Model file for the job. Use its own axes, mm. A direction names the side the tool comes from. Round coordinates to 2 decimals unless told otherwise and drop trailing zeros. Order: outer loops, then holes, each group sorted by start corner. A loop starts at its lowest first (then second) coordinate and runs counter-clockwise, first axis right, second up. Notation, with made-up numbers: M -16.75,-14 L 29.25,-14 A13 cw 29.25,-1 Z; hole C 2.25,-40 d2. An arc over 180 degrees is marked long. Return JSON: item names as keys, results as strings. Group by question number.
Item 1: Slice it at A-A on z = -24. Write the cut outline in (x, y).
Item 2: Pull direction Z, two halves, no side cores. Call faces 1 (the face through (13, 13.839, -13)), 2 (the face through (15.62, 21.51, -3.47)), 3 (the face through (-1.32, 25.33, -29.97)): pulls with the +Z half, pulls with the -Z half, needs draft (parallel to the pull), parting line crosses it, or undercut.
Item 3: Probe line 1 along Z through (x, y) = (0, 24.75); line 2 along X through (y, z) = (27.75, 7). List the from-to ranges inside material, lowest first.
Item 4: Which spindle directions (+Z, -Z, +X, -X, +Y, -Y) get a long thin tool onto all of the face, cutting with end or side? Do faces 4 (the face through (13, 25.839, -13)), 5 (the face through (-1.32, 13.33, -29.97)). Say none if no direction does.
Item 5: Slice it at B-B on y = 23. Write the cut outline in (x, z).
Item 6: Pin check, flat tips, straight feed: pin 1 Ø3 at (x, y) = (-20, 30.5) entering from -Z; pin 2 Ø12 at (y, z) = (12.5, -14) entering from -X; pin 3 Ø3 at (x, y) = (14, 24) entering from -Z. Stop position of each tip, or through.
from build123d import *

# Parameters (mm, degrees)
LPATTERN1_COUNT    = 7
LPATTERN1_PITCH    = 4
SKETCH3_R          = 19.047367533
CUT_EXTRUDE3_DEPTH = 4


with BuildPart() as part:
    # Sketch1 → Revolve1 (revolve)
    with BuildSketch(Plane(origin=(0, 0, 0), x_dir=(0, 0, -1), z_dir=(1, 0, 0))):
        Polygon((-18, 13.838658872), (-18, 9.838658872), (-30, 9.838658872), (-30, 8.838658872), (-16, 8.838658872), (-16, 13.838658872), align=None)
    revolve1 = revolve(axis=Axis((0, 28.058626224, 0), (0, -1, 0)))

    # LPattern1: Revolve1 ×7
    with Locations(*[(0, i * LPATTERN1_PITCH, 0) for i in range(1, LPATTERN1_COUNT)]):
        add(revolve1)

    # Sketch3 → Cut-Extrude3 (cut)
    with BuildSketch(Plane(origin=(0, 37.838658872, 0), x_dir=(1, 0, 0), z_dir=(0, 1, 0))):
        Circle(SKETCH3_R)
    extrude(amount=-CUT_EXTRUDE3_DEPTH, mode=Mode.SUBTRACT)


solid = part.part
Output values:
{
 "1": {"outline": "M -18,8.84 L 18,8.84 L 18,9.84 L -18,9.84 Z; M -18,12.84 L 18,12.84 L 18,13.84 L -18,13.84 Z; M -18,16.84 L 18,16.84 L 18,17.84 L -18,17.84 Z; M -18,20.84 L 18,20.84 L 18,21.84 L -18,21.84 Z; M -18,24.84 L 18,24.84 L 18,25.84 L -18,25.84 Z; M -18,28.84 L 18,28.84 L 18,29.84 L -18,29.84 Z; M -18,32.84 L 18,32.84 L 18,33.84 L -18,33.84 Z"},
 "2": {"face 1": "needs draft", "face 2": "undercut", "face 3": "parting line crosses it"},
 "3": {"line 1": "-18 to -16, 16 to 18", "line 2": "-16.58 to -14.39, 14.39 to 16.58"},
 "4": {"face 4": "none", "face 5": "+Y, -Y"},
 "5": {"outline": "C 0,0 d36; hole C 0,0 d32"},
 "6": {"pin 1": "z = -23.5", "pin 2": "x = -28.91", "pin 3": "z = -27.15"}
}
